Autodesk Inventor part; units mm, degrees
ref_plane "Work Plane1" through (-188.9125, 0, 0) normal (1, 0, 0) x (0, 1, 0)
ref_plane "YZ Plane" through (0, 0, 0) normal (1, 0, 0) x (0, 1, 0)
ref_plane "XZ Plane" through (0, 0, 0) normal (0, 1, 0) x (-1, 0, 0)
ref_plane "Work Plane1" through (-188.9125, 0, 0) normal (1, 0, 0) x (0, 1, 0)
sketch "Sketch1" plane through (-188.9125, 0, 0) normal (1, 0, 0) x (0, 1, 0)
  line L0 (-22.5, -5) -> (-16.5, -5)
  line L1 (-16.5, -5) -> (-16.5, -10.05)
  line L2 (-16.5, -10.05) -> (-11.9175, -10.05)
  line L3 (-11.9175, -10.05) -> (-9.3675, -7.5)
  line L4 (-9.3675, -7.5) -> (-9.3675, -3.5)
  arc A0 (-9.3675, 3.5) -> (-9.3675, -3.5) centre (0, 0) ccw
  line L5 (-9.3675, 3.5) -> (-9.3675, 7.5)
  line L6 (-9.3675, 7.5) -> (-11.9175, 10.05)
  line L7 (-11.9175, 10.05) -> (-16.5, 10.05)
  line L8 (-16.5, 10.05) -> (-16.5, 5)
  line L9 (-22.5, 5) -> (-16.5, 5)
  line L10 (-22.5, 5) -> (-22.5, 19.5)
  arc A1 (-19.5, 22.5) -> (-22.5, 19.5) centre (-19.5, 19.5) ccw
  line L11 (-19.5, 22.5) -> (-5, 22.5)
  line L12 (-5, 22.5) -> (-5, 16.5)
  line L13 (-5, 16.5) -> (-10.05, 16.5)
  line L14 (-10.05, 16.5) -> (-10.05, 11.9175)
  line L15 (-10.05, 11.9175) -> (-7.5, 9.3675)
  line L16 (-7.5, 9.3675) -> (-3.5, 9.3675)
  arc A2 (3.5, 9.3675) -> (-3.5, 9.3675) centre (0, 0) ccw
  line L17 (3.5, 9.3675) -> (7.5, 9.3675)
  line L18 (7.5, 9.3675) -> (10.05, 11.9175)
  line L19 (10.05, 11.9175) -> (10.05, 16.5)
  line L20 (10.05, 16.5) -> (5, 16.5)
  line L21 (5, 22.5) -> (5, 16.5)
  line L22 (5, 22.5) -> (19.5, 22.5)
  arc A3 (22.5, 19.5) -> (19.5, 22.5) centre (19.5, 19.5) ccw
  line L23 (22.5, 19.5) -> (22.5, 5)
  line L24 (22.5, 5) -> (16.5, 5)
  line L25 (16.5, 5) -> (16.5, 10.05)
  line L26 (16.5, 10.05) -> (11.9175, 10.05)
  line L27 (11.9175, 10.05) -> (9.3675, 7.5)
  line L28 (9.3675, 7.5) -> (9.3675, 3.5)
  arc A4 (9.3675, -3.5) -> (9.3675, 3.5) centre (0, 0) ccw
  line L29 (9.3675, -3.5) -> (9.3675, -7.5)
  line L30 (9.3675, -7.5) -> (11.9175, -10.05)
  line L31 (11.9175, -10.05) -> (16.5, -10.05)
  line L32 (16.5, -10.05) -> (16.5, -5)
  line L33 (22.5, -5) -> (16.5, -5)
  line L34 (22.5, -5) -> (22.5, -19.5)
  arc A5 (19.5, -22.5) -> (22.5, -19.5) centre (19.5, -19.5) ccw
  line L35 (19.5, -22.5) -> (5, -22.5)
  line L36 (5, -22.5) -> (5, -16.5)
  line L37 (5, -16.5) -> (10.05, -16.5)
  line L38 (10.05, -16.5) -> (10.05, -11.9175)
  line L39 (10.05, -11.9175) -> (7.5, -9.3675)
  line L40 (7.5, -9.3675) -> (3.5, -9.3675)
  arc A6 (-3.5, -9.3675) -> (3.5, -9.3675) centre (0, 0) ccw
  line L41 (-3.5, -9.3675) -> (-7.5, -9.3675)
  line L42 (-7.5, -9.3675) -> (-10.05, -11.9175)
  line L43 (-10.05, -11.9175) -> (-10.05, -16.5)
  line L44 (-10.05, -16.5) -> (-5, -16.5)
  line L45 (-5, -22.5) -> (-5, -16.5)
  line L46 (-5, -22.5) -> (-19.5, -22.5)
  arc A7 (-22.5, -19.5) -> (-19.5, -22.5) centre (-19.5, -19.5) ccw
  line L47 (-22.5, -19.5) -> (-22.5, -5)
  arc A8 (0, 5) -> (0, -5) centre (0, 0) ccw
  arc A9 (0, -5) -> (0, 5) centre (0, 0) ccw
  arc A10 (13.05, -12.05) -> (12.05, -13.05) centre (13.05, -13.05) ccw
  line L48 (12.05, -13.05) -> (12.05, -18.5)
  line L49 (12.05, -18.5) -> (7, -18.5)
  line L50 (7, -18.5) -> (7, -20.5)
  line L51 (7, -20.5) -> (19.5, -20.5)
  arc A11 (19.5, -20.5) -> (20.5, -19.5) centre (19.5, -19.5) ccw
  line L52 (20.5, -19.5) -> (20.5, -7)
  line L53 (20.5, -7) -> (18.5, -7)
  line L54 (18.5, -7) -> (18.5, -12.05)
  line L55 (18.5, -12.05) -> (13.05, -12.05)
  arc A12 (-20.5, -19.5) -> (-19.5, -20.5) centre (-19.5, -19.5) ccw
  line L56 (-19.5, -20.5) -> (-7, -20.5)
  line L57 (-7, -20.5) -> (-7, -18.5)
  line L58 (-7, -18.5) -> (-12.05, -18.5)
  line L59 (-12.05, -18.5) -> (-12.05, -13.05)
  arc A13 (-12.05, -13.05) -> (-13.05, -12.05) centre (-13.05, -13.05) ccw
  line L60 (-13.05, -12.05) -> (-18.5, -12.05)
  line L61 (-18.5, -12.05) -> (-18.5, -7)
  line L62 (-18.5, -7) -> (-20.5, -7)
  line L63 (-20.5, -7) -> (-20.5, -19.5)
  arc A14 (-19.5, 20.5) -> (-20.5, 19.5) centre (-19.5, 19.5) ccw
  line L64 (-20.5, 19.5) -> (-20.5, 7)
  line L65 (-20.5, 7) -> (-18.5, 7)
  line L66 (-18.5, 7) -> (-18.5, 12.05)
  line L67 (-18.5, 12.05) -> (-13.05, 12.05)
  arc A15 (-13.05, 12.05) -> (-12.05, 13.05) centre (-13.05, 13.05) ccw
  line L68 (-12.05, 13.05) -> (-12.05, 18.5)
  line L69 (-12.05, 18.5) -> (-7, 18.5)
  line L70 (-7, 18.5) -> (-7, 20.5)
  line L71 (-7, 20.5) -> (-19.5, 20.5)
  line L72 (7, 18.5) -> (12.05, 18.5)
  line L73 (12.05, 18.5) -> (12.05, 13.05)
  arc A16 (12.05, 13.05) -> (13.05, 12.05) centre (13.05, 13.05) ccw
  line L74 (13.05, 12.05) -> (18.5, 12.05)
  line L75 (18.5, 12.05) -> (18.5, 7)
  line L76 (18.5, 7) -> (20.5, 7)
  line L77 (20.5, 7) -> (20.5, 19.5)
  arc A17 (20.5, 19.5) -> (19.5, 20.5) centre (19.5, 19.5) ccw
  line L78 (19.5, 20.5) -> (7, 20.5)
  line L79 (7, 20.5) -> (7, 18.5)
  line L80 (5, -22.5) -> (19.5, -22.5)
  line L81 (19.5, -20.5) -> (7, -20.5)
  line L82 (7, -20.5) -> (7, -18.5)
  line L83 (7, -18.5) -> (12.05, -18.5)
  line L84 (12.05, -18.5) -> (12.05, -13.05)
  line L85 (18.5, -12.05) -> (13.05, -12.05)
  line L86 (18.5, -12.05) -> (18.5, -7)
  line L87 (18.5, -7) -> (20.5, -7)
  line L88 (20.5, -7) -> (20.5, -19.5)
  line L89 (22.5, -19.5) -> (22.5, -5)
  line L90 (22.5, -5) -> (16.5, -5)
  line L91 (11.9175, -10.05) -> (16.5, -10.05)
  line L92 (16.5, -10.05) -> (16.5, -5)
  line L93 (11.9175, -10.05) -> (9.3675, -7.5)
  line L94 (7.5, -9.3675) -> (10.05, -11.9175)
  line L95 (10.05, -11.9175) -> (10.05, -16.5)
  line L96 (10.05, -16.5) -> (5, -16.5)
  line L97 (5, -22.5) -> (5, -16.5)
  line L98 (7.5, -9.3675) -> (3.5, -9.3675)
  line L99 (9.3675, -7.5) -> (9.3675, -3.5)
  line L100 (9.3675, 3.5) -> (9.3675, 7.5)
  line L101 (9.3675, 7.5) -> (11.9175, 10.05)
  line L102 (11.9175, 10.05) -> (16.5, 10.05)
  line L103 (16.5, 10.05) -> (16.5, 5)
  line L104 (16.5, 5) -> (22.5, 5)
  line L105 (22.5, 5) -> (22.5, 19.5)
  line L106 (20.5, 19.5) -> (20.5, 7)
  line L107 (18.5, 7) -> (20.5, 7)
  line L108 (18.5, 7) -> (18.5, 12.05)
  line L109 (18.5, 12.05) -> (13.05, 12.05)
  line L110 (12.05, 13.05) -> (12.05, 18.5)
  line L111 (12.05, 18.5) -> (7, 18.5)
  line L112 (7, 18.5) -> (7, 20.5)
  line L113 (7, 20.5) -> (19.5, 20.5)
  line L114 (19.5, 22.5) -> (5, 22.5)
  line L115 (5, 22.5) -> (5, 16.5)
  line L116 (5, 16.5) -> (10.05, 16.5)
  line L117 (10.05, 16.5) -> (10.05, 11.9175)
  line L118 (10.05, 11.9175) -> (7.5, 9.3675)
  line L119 (7.5, 9.3675) -> (3.5, 9.3675)
  line L120 (-3.5, 9.3675) -> (-7.5, 9.3675)
  line L121 (-7.7267, 9.5942) -> (-10.05, 11.9175)
  line L122 (-10.05, 11.9175) -> (-10.05, 16.5)
  line L123 (-10.05, 16.5) -> (-5, 16.5)
  line L124 (-5, 16.5) -> (-5, 22.5)
  line L125 (-19.5, 22.5) -> (-5, 22.5)
  line L126 (-7, 20.5) -> (-19.5, 20.5)
  line L127 (-7, 20.5) -> (-7, 18.5)
  line L128 (-7, 18.5) -> (-12.05, 18.5)
  line L129 (-12.05, 18.5) -> (-12.05, 13.05)
  line L130 (-13.05, 12.05) -> (-18.5, 12.05)
  line L131 (-18.5, 12.05) -> (-18.5, 7)
  line L132 (-18.5, 7) -> (-20.5, 7)
  line L133 (-20.5, 7) -> (-20.5, 19.5)
  line L134 (-22.5, 19.5) -> (-22.5, 5)
  line L135 (-22.5, 5) -> (-16.5, 5)
  line L136 (-16.5, 5) -> (-16.5, 10.05)
  line L137 (-11.9175, 10.05) -> (-16.5, 10.05)
  line L138 (-11.9175, 10.05) -> (-9.3675, 7.5)
  line L139 (-9.3675, 7.5) -> (-9.3675, 3.5)
  line L140 (-9.3675, -3.5) -> (-9.3675, -7.5)
  line L141 (-9.3675, -7.5) -> (-11.9175, -10.05)
  line L142 (-11.9175, -10.05) -> (-16.5, -10.05)
  line L143 (-16.5, -10.05) -> (-16.5, -5)
  line L144 (-16.5, -5) -> (-22.5, -5)
  line L145 (-22.5, -5) -> (-22.5, -19.5)
  line L146 (-20.5, -7) -> (-20.5, -19.5)
  line L147 (-20.5, -7) -> (-18.5, -7)
  line L148 (-18.5, -7) -> (-18.5, -12.05)
  line L149 (-18.5, -12.05) -> (-13.05, -12.05)
  line L150 (-12.05, -13.05) -> (-12.05, -18.5)
  line L151 (-12.05, -18.5) -> (-7, -18.5)
  line L152 (-7, -18.5) -> (-7, -20.5)
  line L153 (-7, -20.5) -> (-19.5, -20.5)
  line L154 (-19.5, -22.5) -> (-5, -22.5)
  line L155 (-5, -22.5) -> (-5, -16.5)
  line L156 (-5, -16.5) -> (-10.05, -16.5)
  line L157 (-10.05, -16.5) -> (-10.05, -11.9175)
  line L158 (-7.5, -9.3675) -> (-10.05, -11.9175)
  line L159 (-7.5, -9.3675) -> (-3.5, -9.3675)
  arc A18 (-20.5, -19.5) -> (-19.5, -20.5) centre (-19.5, -19.5) ccw
  arc A19 (-22.5, -19.5) -> (-19.5, -22.5) centre (-19.5, -19.5) ccw
  arc A20 (-12.05, -13.05) -> (-13.05, -12.05) centre (-13.05, -13.05) ccw
  circle A21 centre (0, 0) radius 5
  arc A22 (-13.05, 12.05) -> (-12.05, 13.05) centre (-13.05, 13.05) ccw
  arc A23 (-19.5, 20.5) -> (-20.5, 19.5) centre (-19.5, 19.5) ccw
  arc A24 (-19.5, 22.5) -> (-22.5, 19.5) centre (-19.5, 19.5) ccw
  arc A25 (12.05, 13.05) -> (13.05, 12.05) centre (13.05, 13.05) ccw
  arc A26 (20.5, 19.5) -> (19.5, 20.5) centre (19.5, 19.5) ccw
  arc A27 (22.5, 19.5) -> (19.5, 22.5) centre (19.5, 19.5) ccw
  arc A28 (13.05, -12.05) -> (12.05, -13.05) centre (13.05, -13.05) ccw
  arc A29 (19.5, -20.5) -> (20.5, -19.5) centre (19.5, -19.5) ccw
  arc A30 (19.5, -22.5) -> (22.5, -19.5) centre (19.5, -19.5) ccw
  arc A31 (-3.5, -9.3675) -> (3.5, -9.3675) centre (0, 0) ccw
  arc A32 (9.3675, -3.5) -> (9.3675, 3.5) centre (0, 0) ccw
  arc A33 (3.5, 9.3675) -> (-3.5, 9.3675) centre (0, 0) ccw
  arc A34 (-9.3675, 3.5) -> (-9.3675, -3.5) centre (0, 0) ccw
extrude "BOSCH, 45X45" add sketch "Sketch1" along normal blind 945
properties part number "BAR, EXTRUDED ALUM, 45MMX45MM, BOSCH" material "Aluminum, 6061-T6"
Geometry check sheet. Reference: the model listing, model coordinates, mm. Coordinates: 2 decimals unless noted, no trailing zeros. Answer as a JSON object with one key per item and string values. Group by question number.
Item 1: Sectioned sample at A-A, the plane x = 412.5. Give the number of separate pieces and of enclosed holes in the cut face, and give its area (3 significant figures).
Item 2: Scan lines: probe 1 along Z at (x, y) = (96, -17); probe 2 along Z at (x, y) = (539, 12); probe 3 along Y at (x, z) = (572, -14.5). Record each from-to range of solid material in increasing order.
Item 3: Depth check by flat-ended pin: pin 1 Ø2 at (y, z) = (-8.5, 14) entering from +X. Enter the tip coordinate at first touch or a pass-through.
Resolved:
{
 "1": {"separate pieces": "1", "enclosed holes": "5", "area": "798 mm^2"},
 "2": {"probe 1": "-22.5 to -20.5, -12.05 to -5, 5 to 12.05, 20.5 to 22.5", "probe 2": "-22.5 to -20.5, -18.5 to -10.05, 10.05 to 18.5, 20.5 to 22.5", "probe 3": "-22.5 to -20.5, -12.05 to -10.05, 10.05 to 12.05, 20.5 to 22.5"},
 "3": {"pin 1": "through"}
}
